Geometry check sheet. Reference: drawing and pictorial views, mm from the part's lowest x, y, z. A direction names the side the tool comes from. Round coordinates to 2 decimals unless told otherwise and drop trailing zeros. Loops run counter-clockwise (first coordinate to the right, second up) from the corner with the lowest first, then second, coordinate; pieces in that order, holes last. Notation, with made-up numbers: (-22.75, -34) -> (-8.75, -34) arc R17 ccw to (-8.75, -10) -> close; hole circle Ø2 at (3.25, 8.5). An arc over 180 degrees is marked (long way). Use one line per item in the form item = value. Start each with the question number.
(1) Sectioned sample at D-D (z = 128). Record the cut outline in (x, y).
(2) Material ranges on probe 1 along Y at (x, z) = (163.5, 46); probe 2 along X at (y, z) = (149, 193), recorded low to high. Write a range as [from, to].
(3) Sectioned sample at A-A (z = 57). Record the cut outline in (x, y), and give its area (3 significant figures).
(4) Set-up check for the marked faces 4, 5, 6 and 7: record each of +Z, -Z, +X, -X, +Y, -Y from which the full face is reachable in a straight line by a thin tool's end or side.
(5) Sectioned sample at B-B (y = 126.5). Record the cut outline in (x, z).
(6) Go/stop test with flat-tipped pins: pin 1 (19 mm diameter, centred on x = 58, y = 130.5, fed in from +Z); pin 2 (23 mm diameter, centred on x = 155, z = 86, fed in from +Y); pin 3 (5 mm diameter, centred on x = 78, y = 187, fed in from +Z). Record where each tip stops, or that it passes through.
(7) Sectioned sample at C-C (x = 135). Record the cut outline in (y, z), and give its area (3 significant figures).
(8) Draft check along Y on the marked faces 1, 2 and 3. Enter one of: released by +Y, released by -Y, zero draft, split by the parting line, or undercut.
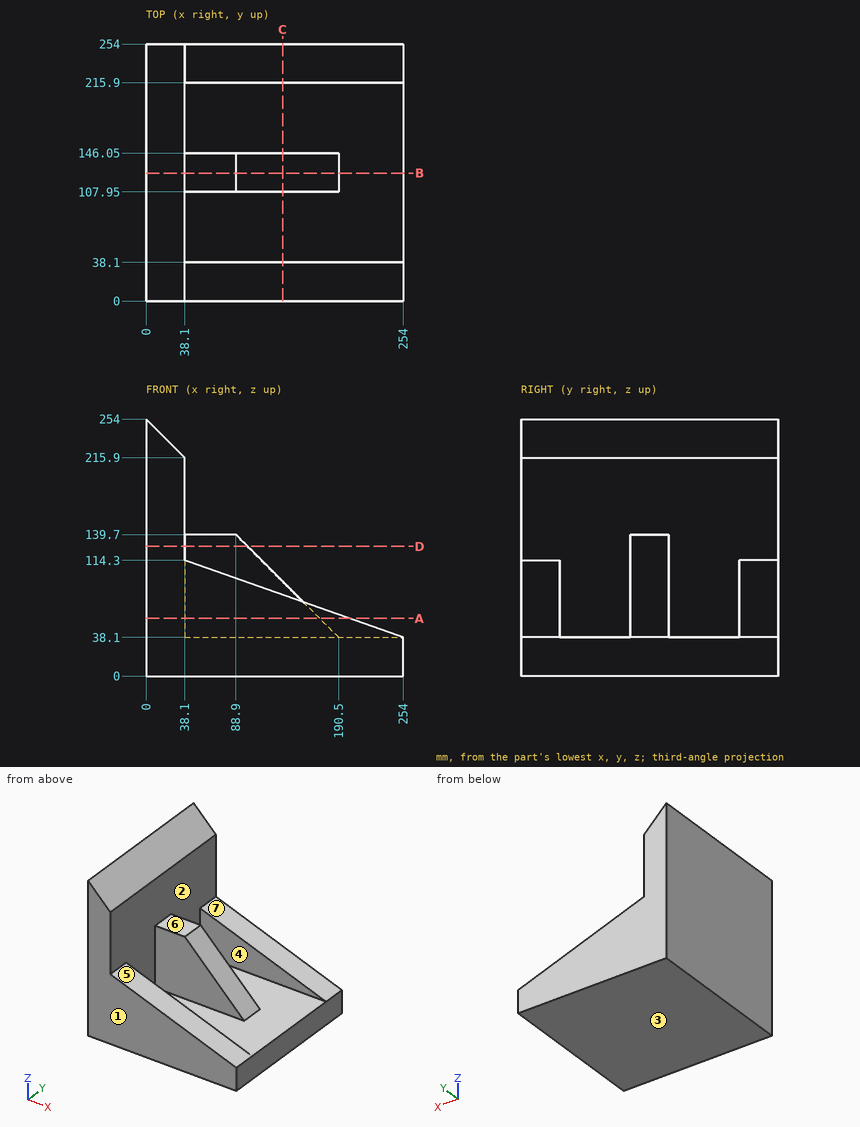
Checks:
q1.outline = (0, 0) -> (38.1, 0) -> (38.1, 107.95) -> (100.6, 107.95) -> (100.6, 146.05) -> (38.1, 146.05) -> (38.1, 254) -> (0, 254) -> close
q2.probe_1 = [0, 38.1], [107.95, 146.05], [215.9, 254]
q2.probe_2 = [0, 38.1]
q3.outline = (0, 0) -> (200.45, 0) -> (200.45, 38.1) -> (38.1, 38.1) -> (38.1, 107.95) -> (171.6, 107.95) -> (171.6, 146.05) -> (38.1, 146.05) -> (38.1, 215.9) -> (200.45, 215.9) -> (200.45, 254) -> (0, 254) -> close
q3.area = 27,100 mm2
q4.face_4 = +Z, +X
q4.face_5 = +Z, +X, -Y
q4.face_6 = +Z, +X, +Y, -Y
q4.face_7 = +Z, +X, +Y
q5.outline = (0, 0) -> (254, 0) -> (254, 38.1) -> (190.5, 38.1) -> (88.9, 139.7) -> (38.1, 139.7) -> (38.1, 215.9) -> (0, 254) -> close
q6.pin_1 = 139.7
q6.pin_2 = 146.05
q6.pin_3 = 38.1
q7.outline = (0, 0) -> (254, 0) -> (254, 80.1) -> (215.9, 80.1) -> (215.9, 38.1) -> (146.05, 38.1) -> (146.05, 93.6) -> (107.95, 93.6) -> (107.95, 38.1) -> (38.1, 38.1) -> (38.1, 80.1) -> (0, 80.1) -> close
q7.area = 15,000 mm2
q8.face_1 = released by -Y
q8.face_2 = undercut
q8.face_3 = zero draft
